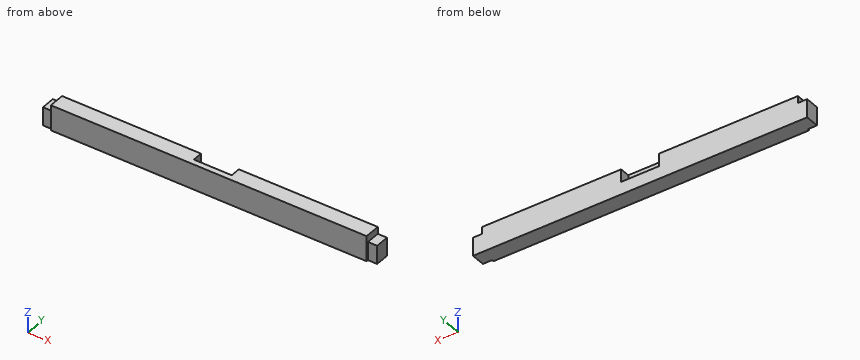
from build123d import *

# Parameters (mm, degrees)
SKETCH1_W           = 635
SKETCH1_H           = 50.8
BOSS_EXTRUDE1_DEPTH = 31.75
SKETCH2_W           = 36.83
SKETCH2_H           = 27.94
BOSS_EXTRUDE2_DEPTH = 18.542
SKETCH3_W           = 36.83
SKETCH3_H           = 27.94
BOSS_EXTRUDE3_DEPTH = 18.542
SKETCH4_W           = 76.2
SKETCH4_H           = 25.4
CUT_EXTRUDE1_DEPTH  = 20.32


with BuildPart() as part:
    # Sketch1 → Boss-Extrude1 (new body)
    with BuildSketch(Plane(origin=(0, 0, 0), x_dir=(1, 0, 0), z_dir=(0, 1, 0))):
        with Locations((317.5, 25.4)):
            Rectangle(SKETCH1_W, SKETCH1_H)
    extrude(amount=BOSS_EXTRUDE1_DEPTH)

    # Sketch2 → Boss-Extrude2 (add)
    with BuildSketch(Plane(origin=(635, 0, 0), x_dir=(0, 0, -1), z_dir=(1, 0, 0))):
        with Locations((32.385, 17.78)):
            Rectangle(SKETCH2_W, SKETCH2_H)
    extrude(amount=BOSS_EXTRUDE2_DEPTH)

    # Sketch3 → Boss-Extrude3 (add)
    with BuildSketch(Plane.ZY):
        with Locations((-32.385, 17.78)):
            Rectangle(SKETCH3_W, SKETCH3_H)
    extrude(amount=BOSS_EXTRUDE3_DEPTH)

    # Sketch4 → Cut-Extrude1 (cut)
    with BuildSketch(Plane(origin=(0, 31.75, 0), x_dir=(1, 0, 0), z_dir=(0, 1, 0))):
        with Locations((317.5, 12.7)):
            Rectangle(SKETCH4_W, SKETCH4_H)
    extrude(amount=-CUT_EXTRUDE1_DEPTH, mode=Mode.SUBTRACT)


solid = part.part
Could you check a few things on this model? Use its own coordinates, in mm. Give positions to 0.01 mm unless a question says otherwise; leave off trailing zeros. Order: outer loops, then holes, each group sorted by start corner. A loop starts at its lowest first (then second) coordinate and runs counter-clockwise, first axis right, second up. Notation, with made-up numbers: (-20.5, -5) - (24.5, -5) arc R21 cw to (24.5, 17) - close; hole circle Ø6 at (-23.5, 2.5). An arc over 180 degrees is marked (long way). One line per item, written item: value. Start each with the question number.
1. Imagine slicing it at B-B on z = -19.5. List the corners of the cut face in (x, y) for me, plus the area to 3 significant figures.
2. Imagine slicing it at A-A on y = 18. List the corners of the cut face in (x, z) for me.
3. For P1, Ø5.5, axis at x = -5, z = -31.5, coming from the -Y side; P2, Ø6, axis at y = 22, z = -6.5, coming from the -X side; P3, Ø20.5, axis at x = 313, z = -8.5, coming from the +Y side, each with a flat end and sliding along its axis, tell me the tip position at first contact or that it passes through.
4. If I drill on probe 1 along X at (y, z) = (27, -9.5); probe 2 along X at (y, z) = (16, -19); probe 3 along X at (y, z) = (2.5, -3), over which ranges is the centre line in solid material (lowest first)?
Values:
1. outline: (-18.54, 3.81) - (0, 3.81) - (0, 0) - (635, 0) - (635, 3.81) - (653.54, 3.81) - (653.54, 31.75) - (355.6, 31.75) - (355.6, 11.43) - (279.4, 11.43) - (279.4, 31.75) - (-18.54, 31.75) - close
1. area: 19,600 mm²
2. outline: (-18.54, -50.8) - (653.54, -50.8) - (653.54, -13.97) - (635, -13.97) - (635, 0) - (355.6, 0) - (355.6, -25.4) - (279.4, -25.4) - (279.4, 0) - (0, 0) - (0, -13.97) - (-18.54, -13.97) - close
3. P1: y = 3.81
3. P2: x = 0
3. P3: y = 11.43
4. probe 1: 0 to 279.4, 355.6 to 635
4. probe 2: -18.54 to 279.4, 355.6 to 653.54
4. probe 3: 0 to 635
